Geometry check sheet. Reference: drawing and pictorial views, mm from the part's lowest x, y, z. A direction names the side the tool comes from. Round coordinates to 2 decimals unless told otherwise and drop trailing zeros. Write each loop counter-clockwise with the first axis right and the second up, starting at its lowest first coordinate (ties: lowest second). Pieces come first, ordered by that corner, then holes. Notation, with made-up numbers: M 67.25,85.5 L 71.25,85.5 A24 ccw 71.25,119.5 Z; hole C 65.5,71 d11. An arc over 180 degrees is marked long. Use a Markdown table: item, result. Add a question column.
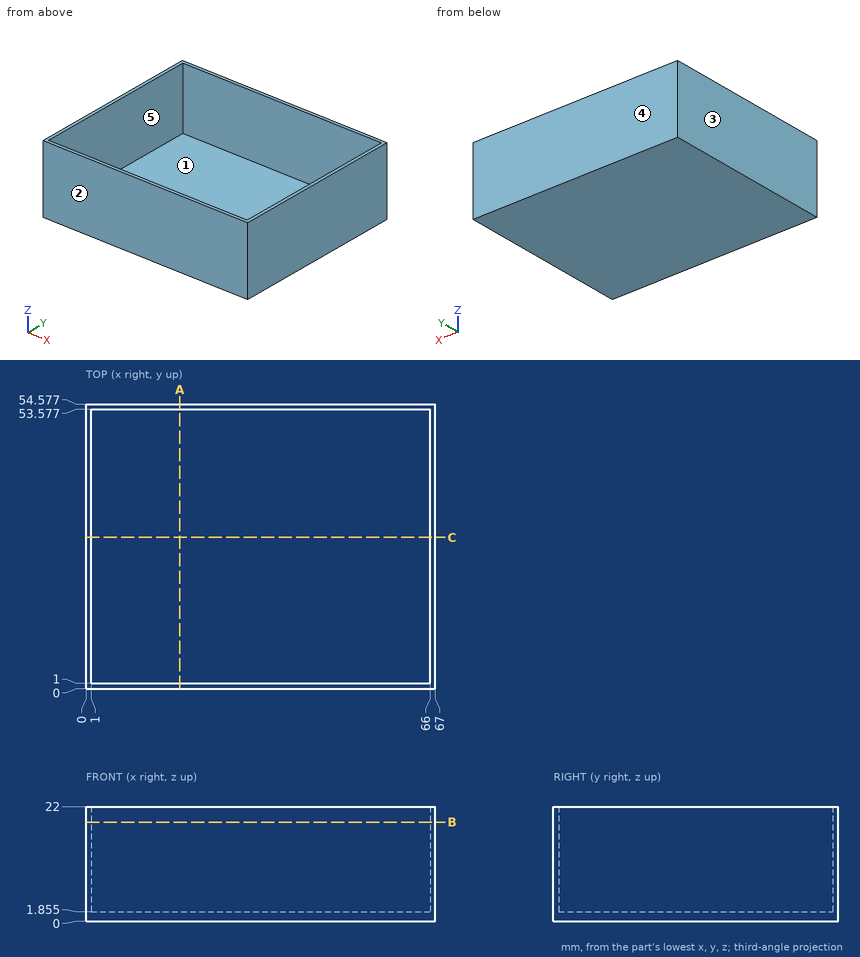
1. Depth check by flat-ended pin: pin 1 Ø10 at (y, z) = (39.5, 19.5) entering from -X; pin 2 Ø1 at (x, y) = (37.5, 39) entering from +Z (3 decimals). Enter the tip coordinate at first touch or a pass-through.
2. Release check for a two-part mould opening along X. For the marked faces 3, 4 and 5 record: +X half, -X half, draft (parallel to the pull), parting line (faces both ways), or undercut.
3. Scan lines: line 1 along Y through (x, z) = (62, 7.75); line 2 along X through (y, z) = (44.5, 17); line 3 along Z through (x, y) = (39, 12) (1 decimal). Record each from-to range of solid material in increasing order. Write a range as from..to.
4. Cross-section at B-B on z = 19. Enter the section's corners in (x, y), plus the area to 3 significant figures.
5. Cross-section at C-C on y = 29. Enter the section's corners in (x, z) (1 decimal).
6. Access from +Z, -Z, +X, -X, +Y, -Y to the whole of each face (thin tool, end or side, straight path). Record for the marked faces 1 and 2.
7. Cross-section at A-A on x = 18. Enter the section's corners in (y, z) (1 decimal).
Answer:
| question | item | result |
|---|---|---|
| 1 | pin 1 | stops at x = 0 |
| 1 | pin 2 | stops at z = 1.855 |
| 2 | face 3 | -X half |
| 2 | face 4 | draft |
| 2 | face 5 | undercut |
| 3 | line 1 | y = 0..1, 53.58..54.58 |
| 3 | line 2 | x = 0..1, 66..67 |
| 3 | line 3 | z = 0..1.9 |
| 4 | outline | M 0,0 L 67,0 L 67,54.58 L 0,54.58 Z; hole M 1,1 L 66,1 L 66,53.58 L 1,53.58 Z |
| 4 | area | 239 mm^2 |
| 5 | outline | M 0,0 L 67,0 L 67,22 L 66,22 L 66,1.9 L 1,1.9 L 1,22 L 0,22 Z |
| 6 | face 1 | +Z |
| 6 | face 2 | +Z, -Z, +X, -X, -Y |
| 7 | outline | M 0,0 L 54.6,0 L 54.6,22 L 53.6,22 L 53.6,1.9 L 1,1.9 L 1,22 L 0,22 Z |
